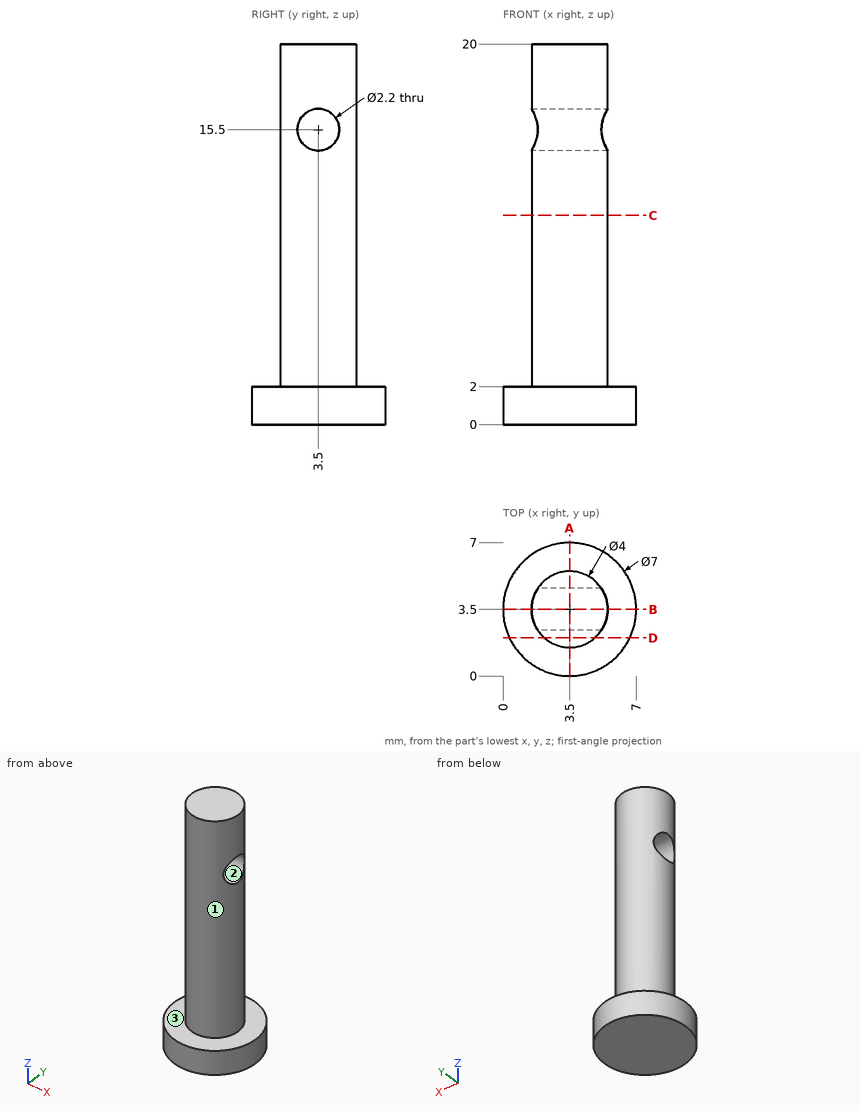
Part print with two shaded views. Sizes in mm from the minimum x, y, z corner. Coordinates: 2 decimals unless noted, no trailing zeros. Loops run counter-clockwise (first coordinate to the right, second up) from the corner with the lowest first, then second, coordinate; pieces in that order, holes last. Notation, with made-up numbers: (55.5, -3) -> (61.5, -3) arc R17 cw to (61.5, 28) -> close; hole circle Ø2 at (42.5, 55). An arc over 180 degrees is marked (long way). Answer as a JSON object with one key per item and string values.
Q1. Probe probe 1 along Z at (x, y) = (3.55, 3.5); probe 2 along Z at (x, y) = (3, 5.5); probe 3 along Y at (x, z) = (3, 15.5). List the from-to ranges inside material, lowest first.
Report:
{"probe 1": "z = 0 to 14.4, 16.6 to 20", "probe 2": "z = 0 to 2", "probe 3": "y = 1.56 to 2.4, 4.6 to 5.44"}
Q2. Pull direction Y, two halves, no side cores. Call the marked faces 1, 2 and 3: released by +Y, released by -Y, zero draft, split by the parting line, or undercut.
Report:
{"face 1": "split by the parting line", "face 2": "undercut", "face 3": "zero draft"}
Q3. Cut at A-A (x = 3.5). List the corners of the cut face in (y, z), and give its area (3 significant figures).
Report:
{"outline": "(0, 0) -> (7, 0) -> (7, 2) -> (5.5, 2) -> (5.5, 20) -> (1.5, 20) -> (1.5, 2) -> (0, 2) -> close; hole circle Ø2.2 at (3.5, 15.5)", "area": "82.2 mm2"}
Q4. Cut at C-C (z = 11). List the corners of the cut face in (x, y), and give its area (3 significant figures).
Report:
{"outline": "circle Ø4 at (3.5, 3.5)", "area": "12.6 mm2"}
Q5. Flat gauge pins, fed straight in: P1, Ø2, axis at y = 3.5, z = 15.5, coming from the -X side; P2, Ø1, axis at y = 5, z = 12, coming from the +X side; P3, Ø1.5, axis at y = 4.5, z = 18, coming from the -X side; P4, Ø3, axis at y = 3.5, z = 10, coming from the +X side. Where does each tip first touch, or does it go through?
Report:
{"P1": "passes through", "P2": "stops at x = 5.23", "P3": "stops at x = 1.52", "P4": "stops at x = 5.5"}
Q6. Cut at D-D (y = 2). List the corners of the cut face in (x, z), and give its area (3 significant figures).
Report:
{"outline": "(0.34, 0) -> (6.66, 0) -> (6.66, 2) -> (4.82, 2) -> (4.82, 20) -> (2.18, 20) -> (2.18, 2) -> (0.34, 2) -> close", "area": "60.3 mm2"}
Q7. Cut at B-B (y = 3.5). List the corners of the cut face in (x, z).
Report:
{"outline": "(0, 0) -> (7, 0) -> (7, 2) -> (5.5, 2) -> (5.5, 14.4) -> (1.5, 14.4) -> (1.5, 2) -> (0, 2) -> close; (1.5, 16.6) -> (5.5, 16.6) -> (5.5, 20) -> (1.5, 20) -> close"}
